Check sheet for the drawn part. Datum: minimum x, y, z corner. Units: mm. Give positions to 0.01 mm unless a question says otherwise; leave off trailing zeros. Order: outer loops, then holes, each group sorted by start corner. A loop starts at its lowest first (then second) coordinate and runs counter-clockwise, first axis right, second up. Notation, with made-up numbers: (-13.75, 78) - (45.25, 78) arc R22 ccw to (45.25, 117) - close; hole circle Ø5 at (24, 71.5). An arc over 180 degrees is marked (long way). Answer as a JSON object with one key per item and string values. Group by question number.
(1) Section check A-A (y = 7). Record the boundary of the cut face in (x, z).
(2) Section check D-D (x = 180). Record the boundary of the cut face in (y, z), then the cut area to 3 significant figures.
(3) Thickness scan on line 1 (Y direction, x = 6, z = 0.95); line 2 (X direction, y = 93, z = 1.15); line 3 (X direction, y = 20, z = 1.1). Record the ranges inside material, lowest first.
(4) Section check B-B (x = 149). Record the boundary of the cut face in (y, z), then the cut area to 3 significant figures.
(5) Section check C-C (z = 1.9). Record the boundary of the cut face in (x, y).
(6) Depth check by flat-ended pin: pin 1 Ø3 at (x, y) = (180, 7) entering from -Z. Enter the tip coordinate at first touch or a pass-through.
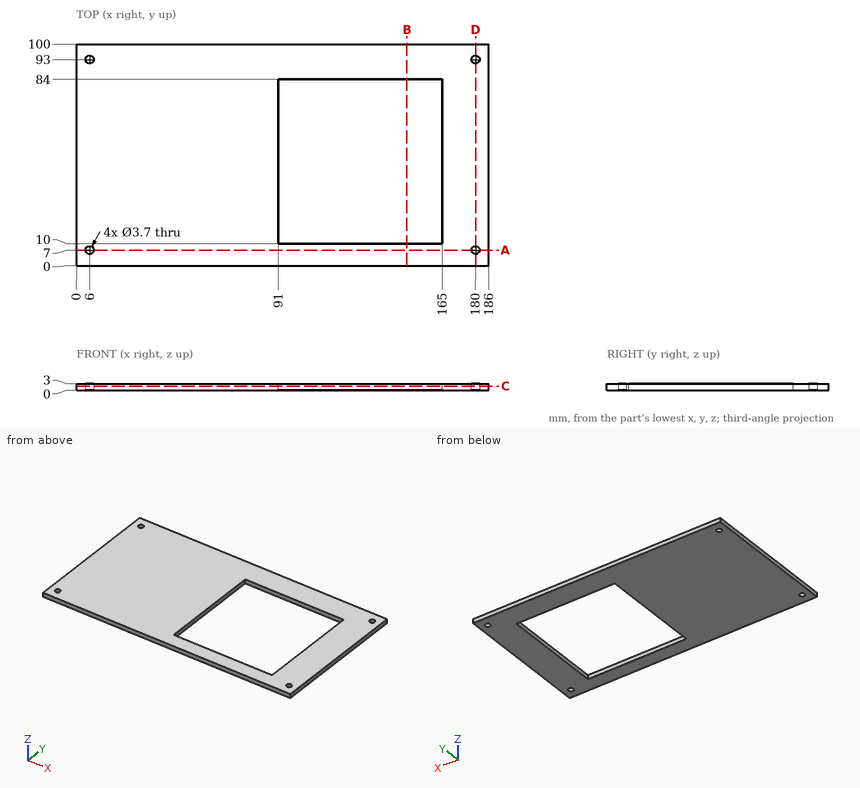
Solutions:
{
 "1": {"outline": "(0, 0) - (4.15, 0) - (4.15, 3) - (0, 3) - close; (7.85, 0) - (178.15, 0) - (178.15, 3) - (7.85, 3) - close; (181.85, 0) - (186, 0) - (186, 3) - (181.85, 3) - close"},
 "2": {"outline": "(0, 0) - (5.15, 0) - (5.15, 3) - (0, 3) - close; (8.85, 0) - (91.15, 0) - (91.15, 3) - (8.85, 3) - close; (94.85, 0) - (100, 0) - (100, 3) - (94.85, 3) - close", "area": "278 mm2"},
 "3": {"line 1": "y = 0 to 5.15, 8.85 to 91.15, 94.85 to 100", "line 2": "x = 0 to 4.15, 7.85 to 178.15, 181.85 to 186", "line 3": "x = 0 to 91, 165 to 186"},
 "4": {"outline": "(0, 0) - (10, 0) - (10, 3) - (0, 3) - close; (84, 0) - (100, 0) - (100, 3) - (84, 3) - close", "area": "78.0 mm2"},
 "5": {"outline": "(0, 0) - (186, 0) - (186, 100) - (0, 100) - close; hole circle Ø3.7 at (6, 7); hole circle Ø3.7 at (6, 93); hole (91, 10) - (165, 10) - (165, 84) - (91, 84) - close; hole circle Ø3.7 at (180, 7); hole circle Ø3.7 at (180, 93)"},
 "6": {"pin 1": "passes through"}
}
